Design review of the part built by this model. Coordinates are the model's own, in mm. Round coordinates to 2 decimals unless told otherwise and drop trailing zeros. Write each loop counter-clockwise with the first axis right and the second up, starting at its lowest first coordinate (ties: lowest second). Pieces come first, ordered by that corner, then holes. Notation, with made-up numbers: (68, -23.5) - (107, -23.5) arc R19 cw to (107, -5.5) - close; hole circle Ø11 at (27, 56). An arc over 180 degrees is marked (long way). Use one line per item in the form item = value.
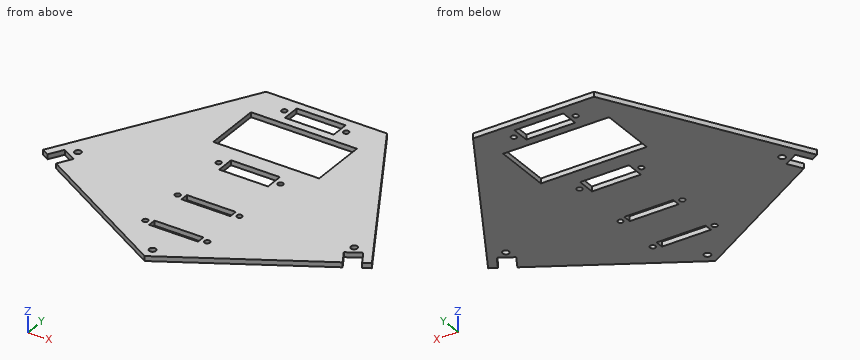
```python
from build123d import *

# Parameters (mm, degrees)
ESQUISSE1_R        = 2
ESQUISSE1_R_2      = 1.65
ESQUISSE1_W        = 65
ESQUISSE1_H        = 35
ESQUISSE1_W_2      = 30
ESQUISSE1_H_2      = 5
ESQUISSE1_H_3      = 11
BOSS_EXTRU_1_DEPTH = 3


with BuildPart() as part:
    # Esquisse1 → Boss.-Extru.1 (new body)
    with BuildSketch(Plane.XY):
        Polygon((37.118802154, 168.871977627), (100.962812921, 58.290907218), (96.632685902, 55.790907218), (91.632685902, 64.451161256), (82.972431864, 59.451161256), (87.972431864, 50.790907218), (0, 0), (-87.972431864, 50.790907218), (-82.972431864, 59.451161256), (-91.632685902, 64.451161256), (-96.632685902, 55.790907218), (-100.962812921, 58.290907218), (-37.118802153, 168.871977627), align=None)
        with Locations((-84.802558883, 66.281288275)):
            Circle(ESQUISSE1_R, mode=Mode.SUBTRACT)
        with Locations((84.802558883, 66.281288275)):
            Circle(ESQUISSE1_R, mode=Mode.SUBTRACT)
        with Locations((-19, 97.371977627)):
            Circle(ESQUISSE1_R_2, mode=Mode.SUBTRACT)
        with Locations((19, 97.371977627)):
            Circle(ESQUISSE1_R_2, mode=Mode.SUBTRACT)
        with Locations((19, 158.371977627)):
            Circle(ESQUISSE1_R_2, mode=Mode.SUBTRACT)
        with Locations((-19, 158.371977627)):
            Circle(ESQUISSE1_R_2, mode=Mode.SUBTRACT)
        with Locations((-19, 59.371977627)):
            Circle(ESQUISSE1_R_2, mode=Mode.SUBTRACT)
        with Locations((0, 7.342924489)):
            Circle(ESQUISSE1_R, mode=Mode.SUBTRACT)
        with Locations((19, 59.371977627)):
            Circle(ESQUISSE1_R_2, mode=Mode.SUBTRACT)
        with Locations((19, 29.371977627)):
            Circle(ESQUISSE1_R_2, mode=Mode.SUBTRACT)
        with Locations((-19, 29.371977627)):
            Circle(ESQUISSE1_R_2, mode=Mode.SUBTRACT)
        with Locations((0, 130.371977627)):
            Rectangle(ESQUISSE1_W, ESQUISSE1_H, mode=Mode.SUBTRACT)
        with Locations((0, 59.371977627)):
            Rectangle(ESQUISSE1_W_2, ESQUISSE1_H_2, mode=Mode.SUBTRACT)
        with Locations((0, 29.371977627)):
            Rectangle(ESQUISSE1_W_2, ESQUISSE1_H_2, mode=Mode.SUBTRACT)
        with Locations((0, 97.371977627)):
            Rectangle(ESQUISSE1_W_2, ESQUISSE1_H_3, mode=Mode.SUBTRACT)
        with Locations((0, 158.371977627)):
            Rectangle(ESQUISSE1_W_2, ESQUISSE1_H_3, mode=Mode.SUBTRACT)
    extrude(amount=BOSS_EXTRU_1_DEPTH)


solid = part.part
```
Q1. We need section A-A on x = -23. Write out the cut boundary in (y, z).
Calculated:
outline = (13.28, 0) - (112.87, 0) - (112.87, 3) - (13.28, 3) - close; (147.87, 0) - (168.87, 0) - (168.87, 3) - (147.87, 3) - close
Q2. For P1, Ø0.9, axis at x = -8.5, z = 1, coming from the -Y side; P2, Ø3, axis at x = -84.8, y = 66.28, coming from the +Z side (3 decimals); P3, Ø1.5, axis at x = 6, z = 1.5, coming from the -Y side; P4, Ø1.5, axis at x = -72.5, z = 1, coming from the +Y side, all flat-tipped, find the tip position at first contact; note any pin that passes through.
Calculated:
P1 = 4.65
P2 = through
P3 = 3.03
P4 = 108.89
Q3. To check wall thickness, follow line 1 along Y through (x, z) = (13.5, 0.25); line 2 along X through (y, z) = (65, 1.9); line 3 along X through (y, z) = (57, 0.95). State the ranges of each line that lie inside material, in increasing order. Write a range as from..to.
Calculated:
line_1 = 7.79..26.87, 31.87..56.87, 61.87..91.87, 102.87..112.87, 147.87..152.87, 163.87..168.87
line_2 = -97.09..-86.34, -83.27..83.27, 86.34..97.09
line_3 = -98.73..-95.93, -84.39..-15, 15..84.39, 95.93..98.73
Q4. We need section B-B on x = 70. Write out the cut boundary in (y, z), then the cut area to 3 significant figures.
Calculated:
outline = (40.41, 0) - (111.92, 0) - (111.92, 3) - (40.41, 3) - close
area = 215 mm2
Q5. We need section D-D on y = 13. Write out the cut boundary in (x, z).
Calculated:
outline = (-22.52, 0) - (22.52, 0) - (22.52, 3) - (-22.52, 3) - close
Q6. We need section C-C on z = 2.5. State how many separate pieces and enclosed holes the cut face has, then the cut area to 3 significant figures.
Calculated:
separate_pieces = 1
enclosed_holes = 16
area = 17,600 mm2
